```python
from build123d import *
from build123d.topology import SkipClean

# Parameters (mm, degrees)
SKETCH1_R                            = 31.5
BOSS_EXTRUDE1_DEPTH                  = 3.5
SKETCH2_R                            = 1.5
CUT_EXTRUDE1_DEPTH                   = 4
CIRPATTERN1_COUNT                    = 6
SKETCH3_W                            = 30
SKETCH3_H                            = 7
SKETCH3_R                            = 1.5
BOSS_EXTRUDE2_DEPTH                  = 6
BOSS_EXTRUDE2_DIRECTION_2_REACH      = 77.498
BOSS_EXTRUDE2_DIRECTION_2_END_RADIUS = 31.5
SKETCH6_W                            = 26.400196428
SKETCH6_H                            = 7
SKETCH6_R                            = 1.5
BOSS_EXTRUDE3_DEPTH                  = 6
BOSS_EXTRUDE4_REACH                  = 83.142
SKETCH7_W                            = 10.400196428
SKETCH7_H                            = 7


with BuildPart() as part:
    # Sketch1 → Boss-Extrude1 (new, symmetric)
    with BuildSketch(Plane(origin=(0, 0, 0), x_dir=(1, 0, 0), z_dir=(0, 1, 0))):
        with Locations(Location((0, 0, 0), (0, 0, 270))):
            Circle(SKETCH1_R)
    extrude(amount=BOSS_EXTRUDE1_DEPTH, both=True)

    # Sketch2 → Cut-Extrude1 (cut)
    with BuildSketch(Plane(origin=(27.279800219, 0, -15.75), x_dir=(-0.499999999999998, 0, -0.8660254037844398), z_dir=(0.8660254037844399, 0, -0.49999999999999806))):
        Circle(SKETCH2_R)
    cut_extrude1 = extrude(amount=-CUT_EXTRUDE1_DEPTH, mode=Mode.SUBTRACT)

    # CirPattern1: Cut-Extrude1 ×6 about axis
    cirpattern1_axis = Axis((0, 0, 0), (0, 1, 0))
    for i in range(1, CIRPATTERN1_COUNT):
        add(cut_extrude1.rotate(cirpattern1_axis, i * 360 / CIRPATTERN1_COUNT), mode=Mode.SUBTRACT)


with BuildPart() as body_2:
    # Sketch3 → Boss-Extrude2 (new body)
    with BuildSketch(Plane(origin=(27.279800219, 0, -15.75), x_dir=(-0.499999999999998, 0, -0.8660254037844398), z_dir=(0.8660254037844399, 0, -0.49999999999999806))):
        with Locations((5, 0)):
            Rectangle(SKETCH3_W, SKETCH3_H)
        Circle(SKETCH3_R, mode=Mode.SUBTRACT)
    extrude(amount=BOSS_EXTRUDE2_DEPTH)

    # Boss-Extrude2 direction 2: up to this cylinder (the profile starts outside it)
    with SkipClean():  # the faces are left unmerged after this step: merging them gives an invalid solid
        boss_extrude2_direction_2_end = Plane(origin=(0, 0, 0), z_dir=(0, 1, 0)) * Cylinder(BOSS_EXTRUDE2_DIRECTION_2_END_RADIUS, 218.996, mode=Mode.PRIVATE)
        # Sketch3 → Boss-Extrude2 direction 2 (add, up to the surface)
        with BuildSketch(Plane(origin=(27.279800219, 0, -15.75), x_dir=(-0.499999999999998, 0, -0.8660254037844398), z_dir=(0.8660254037844399, 0, -0.49999999999999806)), mode=Mode.PRIVATE) as boss_extrude2_direction_2_sk1:
            with Locations((5, 0)):
                Rectangle(SKETCH3_W, SKETCH3_H)
            Circle(SKETCH3_R, mode=Mode.SUBTRACT)
        boss_extrude2_direction_2_tool1 = extrude(boss_extrude2_direction_2_sk1.sketch, amount=-BOSS_EXTRUDE2_DIRECTION_2_REACH, mode=Mode.PRIVATE) - boss_extrude2_direction_2_end
        add(boss_extrude2_direction_2_tool1.solids().sort_by_distance((24.692719, 0, -20.230956))[0])
        add(boss_extrude2_direction_2_tool1.solids().sort_by_distance((24.692719, 0, -20.230956))[1])

    # Sketch7 → Boss-Extrude4 (add, up to next)
    with BuildSketch(Plane.XY.offset(-40.383857754), mode=Mode.PRIVATE) as boss_extrude4_sk1:
        with Locations((24.275854428, 0)):
            Rectangle(SKETCH7_W, SKETCH7_H)
    boss_extrude4_tool1 = extrude(boss_extrude4_sk1.sketch, amount=BOSS_EXTRUDE4_REACH, mode=Mode.PRIVATE) - body_2.part


with BuildPart() as body_3:
    # Sketch6 → Boss-Extrude3 (new body)
    with BuildSketch(Plane.XY.offset(-46.383857754)):
        with Locations((24.275854428, 0)):
            Rectangle(SKETCH6_W, SKETCH6_H)
        with Locations((32.475952642, 0)):
            Circle(SKETCH6_R, mode=Mode.SUBTRACT)
        with Locations((16.075756214, 0)):
            Circle(SKETCH6_R, mode=Mode.SUBTRACT)
    extrude(amount=BOSS_EXTRUDE3_DEPTH)


with BuildPart() as body_2_1:
    add(body_2.part)

    add(body_3.part)  # Boss-Extrude4 merges body 3
    add(boss_extrude4_tool1.solids().sort_by_distance((24.275854, 0, -40.383858))[0])


solid = body_2_1.part
```
Read the model definition and answer for the solid it produces. Units are mm, in the model's axes. A direction names the side the tool comes from. Coordinates: 2 decimals unless noted, no trailing zeros. Loops run counter-clockwise (first coordinate to the right, second up) from the corner with the lowest first, then second, coordinate; pieces in that order, holes last. Notation, with made-up numbers: (18.25, -36.75) -> (46.25, -36.75) arc R37 ccw to (46.25, 0.25) -> close; hole circle Ø1 at (12.5, 42.5). An arc over 180 degrees is marked (long way). Return JSON: item names as keys, results as strings.
Item 1: For a pull along Y with two mould halves and no side action, classify faces 1 (the flat face through (24, 3.5, -31)), 2 (the flat face through (19.076, 0, -37)), 3 (the cylindrical face through (30.977, 0.066, -43.426)) as +Y half, -Y half, draft (parallel to the pull), parting line (faces both ways), or undercut.
Answers:
{"face 1": "+Y half", "face 2": "draft", "face 3": "undercut"}
Item 2: Find section D-D (z = -12). Determine the outline of the cut face in (x, y), plus the area to 3 significant figures.
Answers:
{"outline": "(29.12, -3.5) -> (36.37, -3.5) -> (36.37, 3.5) -> (29.12, 3.5) -> close", "area": "50.7 mm2"}
Item 3: Find section B-B (x = 15.5). Determine the outline of the cut face in (y, z).
Answers:
{"outline": "(-3.5, -46.38) -> (-1.39, -46.38) -> (-1.39, -40.38) -> (-3.5, -40.38) -> close; (-3.5, -32.04) -> (3.5, -32.04) -> (3.5, -27.42) -> (-3.5, -27.42) -> close; (1.39, -46.38) -> (3.5, -46.38) -> (3.5, -40.38) -> (1.39, -40.38) -> close"}
Item 4: Find the intervals of material crossed by probe 1 along Z at (x, y) = (28, 3); probe 2 along Y at (x, z) = (31.75, -41); probe 3 along X at (y, z) = (3, -40), in increasing order.
Answers:
{"probe 1": "z = -46.38 to -14.43", "probe 2": "y = -3.5 to -1.31, 1.31 to 3.5", "probe 3": "x = 19.08 to 29.48"}
Item 5: Flat-ended cylindrical pins translate along their axes: P1, Ø3.5, axis at x = 14.5, y = 0, coming from the +Z side; P2, Ø1.8, axis at x = 32.48, y = 0, coming from the +Z side; P3, Ø2, axis at x = 33, y = 1.5, coming from the +Z side. Find the tip coordinate at first contact, or state that the pin passes through.
Answers:
{"P1": "stops at z = -26.98", "P2": "stops at z = -6.69", "P3": "stops at z = -6.93"}
Item 6: For faces 4 (the cylindrical face through (17.506, 0.451, -43.426)), 5 (the cylindrical face through (30.648, 0.066, -15.964)), 6 (the flat face through (14, 0, -40.384)), 7 (the flat face through (34.3, 0, -40.384)), determine the directions among +Z, -Z, +X, -X, +Y, -Y from which every point of the face is accessible in a straight line to the end or side of a thin tool.
Answers:
{"face 4": "-Z", "face 5": "none", "face 6": "-X, +Y, -Y", "face 7": "+X, +Y, -Y"}
Item 7: Find section A-A (y = 1). Determine the outline of the cut face in (x, z), plus the area to 3 significant figures.
Answers:
{"outline": "(11.08, -46.38) -> (14.96, -46.38) -> (14.96, -40.38) -> (11.08, -40.38) -> close; (11.08, -29.49) -> (19.08, -34.11) -> (19.08, -40.38) -> (17.19, -40.38) -> (17.19, -46.38) -> (31.36, -46.38) -> (31.36, -40.38) -> (29.48, -40.38) -> (29.48, -23.95) -> (31.92, -19.72) -> (26.7, -16.71) arc R31.5 cw to start; (27.82, -14.77) -> (33.03, -17.78) -> (37.48, -10.09) -> (30.87, -6.28) arc R31.5 cw to start; (33.59, -46.38) -> (37.48, -46.38) -> (37.48, -40.38) -> (33.59, -40.38) -> close", "area": "439 mm2"}
Item 8: Find section C-C (x = 30.25). Count the separate pieces of the cut face and the enclosed holes in it, plus the area to 3 significant figures.
Answers:
{"separate pieces": "2", "enclosed holes": "1", "area": "131 mm2"}
